Work out the finished part from the listing and answer in its coordinate system (mm). A direction names the side the tool comes from. Round coordinates to 2 decimals unless told otherwise and drop trailing zeros. Loops run counter-clockwise (first coordinate to the right, second up) from the corner with the lowest first, then second, coordinate; pieces in that order, holes last. Notation, with made-up numbers: M 47,25.25 L 74,25.25 A12 cw 74,35.25 Z; hole C -23.75,7 d11. An arc over 180 degrees is marked long. One line per item, written item: value.
```python
from build123d import *

# Parameters (mm, degrees)
F2_W     = 3
F2_H     = 11.5
F3_DEPTH = 25
F5_DEPTH = 15.679571
F6_W     = 15
F6_H     = 3
F7_DEPTH = 2
F8_W     = 3
F8_H     = 3.791901
F9_DEPTH = 5


with BuildPart() as f1:
    # F0 (on Front) → F1 (revolve)
    with BuildSketch(Plane.XZ):
        Polygon((0, 20), (0, 0), (11.5, 0), (17.5, 3), (17.5, 4), (4, 4), (4, 17), (7, 17), (7, 18.5), align=None)
    revolve(axis=Axis((0, 0, 10), (0, 0, -1)))

    # F2 (on Front) → F3 (cut, symmetric)
    with BuildSketch(Plane.XZ):
        with Locations((0, 14.75)):
            Rectangle(F2_W, F2_H)
    extrude(amount=F3_DEPTH, both=True, mode=Mode.SUBTRACT)

    # F4 (on face) → F5 (cut, through all)
    with BuildSketch(Plane.XY.offset(4)):
        with BuildLine():
            ThreePointArc((3.464102, -2), (0, -4), (-3.464102, -2))
            Line((-3.464102, -2), (-11.425484, -2))
            Line((-11.425484, -2), (-11.425484, -9.836984))
            Line((-11.425484, -9.836984), (10.346696, -9.836984))
            Line((10.346696, -9.836984), (10.346696, -2))
            Line((10.346696, -2), (3.464102, -2))
        make_face()
        with BuildLine():
            Line((-11.425484, 9.079754), (-11.425484, 2))
            Line((-11.425484, 2), (-3.464102, 2))
            ThreePointArc((-3.464102, 2), (0, 4), (3.464102, 2))
            Line((3.464102, 2), (10.346696, 2))
            Line((10.346696, 2), (10.346696, 9.079754))
            Line((10.346696, 9.079754), (-11.425484, 9.079754))
        make_face()
    extrude(amount=F5_DEPTH, mode=Mode.SUBTRACT)

    # F6 (on face) → F7 (cut)
    with BuildSketch(Plane(origin=(0, 0, 0), x_dir=(1, 0, 0), z_dir=(0, 0, -1))):
        Rectangle(F6_W, F6_H)
    extrude(amount=-F7_DEPTH, mode=Mode.SUBTRACT)

    # F8 (on face) → F9 (cut, through all)
    with BuildSketch(Plane.XY.offset(9)):
        with Locations((0, 3.104049)):
            Rectangle(F8_W, F8_H)
        with Locations((0, -3.104049)):
            Rectangle(F8_W, F8_H)
    extrude(amount=-F9_DEPTH, mode=Mode.SUBTRACT)


solid = f1.part
```
1) The mould has two halves that part along Z. Classify faces 4 (the face through (5, 0, 17)), 5 (the face through (0, 1.208, 7)), 6 (the face through (0, 2, 0)): +Z half, -Z half, draft (parallel to the pull), parting line (faces both ways), or undercut.
Check values:
face 4: undercut
face 5: draft
face 6: -Z half
2) Each of these flat-tipped pins is pushed along its axis until it touches: pin 1 (8 mm diameter, centred on y = -1.5, z = 14, fed in from -X); pin 2 (1.1 mm diameter, centred on x = 5.5, z = 18.5, fed in from +Y); pin 3 (5 mm diameter, centred on y = 6.5, z = 4, fed in from -X); pin 4 (3 mm diameter, centred on x = -5.5, y = -0.5, fed in from -Z). Where does it stop, or does it pass through?
Check values:
pin 1: x = -7
pin 2: y = 2
pin 3: x = -17.04
pin 4: z = 0
3) Find section B-B (y = 0). Give the vertices of the cut face in (x, z), then the cut area to 3 significant figures.
Check values:
outline: M -17.5,3 L -11.5,0 L -7.5,0 L -7.5,2 L 7.5,2 L 7.5,0 L 11.5,0 L 17.5,3 L 17.5,4 L 4,4 L 4,17 L 7,17 L 7,18.5 L 1.5,19.68 L 1.5,9 L -1.5,9 L -1.5,19.68 L -7,18.5 L -7,17 L -4,17 L -4,4 L -17.5,4 Z
area: 195 mm2
4) Find the intervals of material crossed by probe 1 along X at (y, z) = (-1.5, 11.5); probe 2 along Z at (x, y) = (8, -5); probe 3 along Y at (x, z) = (1, 8), in increasing order. Write a range as from..to.
Check values:
probe 1: -3.71..-1.5, 1.5..3.71
probe 2: 0..4
probe 3: -1.21..1.21
5) Find section A-A (x = 0). Give the vertices of the cut face in (y, z).
Check values:
outline: M -17.5,3 L -11.5,0 L -1.5,0 L -1.5,2 L 1.5,2 L 1.5,0 L 11.5,0 L 17.5,3 L 17.5,4 L 1.21,4 L 1.21,9 L -1.21,9 L -1.21,4 L -17.5,4 Z
6) For faces 1 (the face through (-5, -2, 18)), 2 (the face through (-7.5, 0, 1)), 3 (the face through (-5, 2, 18)), determine the directions among +Z, -Z, +X, -X, +Y, -Y from which every point of the face is accessible in a straight line to the end or side of a thin tool.
Check values:
face 1: +Z, -X, -Y
face 2: -Z
face 3: +Z, -X, +Y
